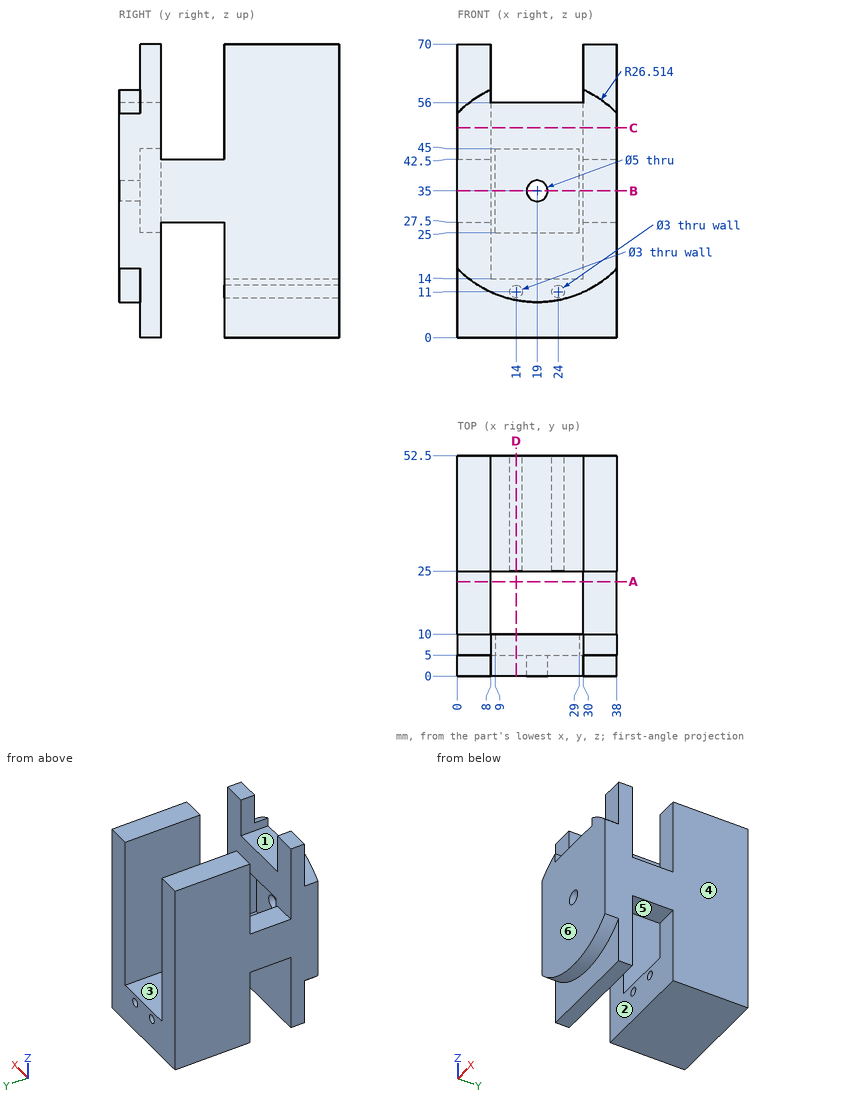
Geometry check sheet. Reference: drawing and pictorial views, mm from the part's lowest x, y, z. A direction names the side the tool comes from. Give positions to 0.01 mm unless a question says otherwise; leave off trailing zeros. Order: outer loops, then holes, each group sorted by start corner. A loop starts at its lowest first (then second) coordinate and runs counter-clockwise, first axis right, second up.
1. Access from +Z, -Z, +X, -X, +Y, -Y to the whole of each face (thin tool, end or side, straight path). Record for the marked faces 1, 2 and 3.
2. Section check C-C, the plane z = 50. Enter the section's corners in (x, y).
3. Section check A-A, the plane y = 22.5. Enter the section's corners in (x, z).
4. Section check D-D, the plane x = 14. Enter the section's corners in (y, z).
5. Thickness scan on L1, parallel to X at y = 33, z = 11; L2, parallel to X at y = 19, z = 38; L3, parallel to Y at x = 2.5, z = 66. Record the ranges inside material, lowest first.
6. Gauge pin test, flat ends, axial feed: pin 1 Ø5 at (x, z) = (34, 51.5) entering from -Y; pin 2 Ø1.5 at (x, z) = (13, 7) entering from -Y; pin 3 Ø4 at (x, y) = (23.5, 7.5) entering from +Z; pin 4 Ø2.5 at (x, z) = (24, 11) entering from +Y. Record the tip position at first contact, or that the pin passes through.
7. Section check B-B, the plane z = 35. Enter the section's corners in (x, y), and give its area (3 significant figures).
8. Release check for a two-part mould opening along Y. For the marked faces 4, 5 and 6 record: pulls with the +Y half, pulls with the -Y half, needs draft (parallel to the pull), parting line crosses it, or undercut.
Values follow:
1. face 1: +Z, +Y, -Y
1. face 2: -Z, +X, -X
1. face 3: +Z, +Y
2. outline: (0, 0) - (38, 0) - (38, 10) - (0, 10) - close; (0, 25) - (8, 25) - (8, 52.5) - (0, 52.5) - close; (30, 25) - (38, 25) - (38, 52.5) - (30, 52.5) - close
3. outline: (0, 27.5) - (8, 27.5) - (8, 42.5) - (0, 42.5) - close; (30, 27.5) - (38, 27.5) - (38, 42.5) - (30, 42.5) - close
4. outline: (0, 8.96) - (5, 8.96) - (5, 0) - (10, 0) - (10, 25) - (5, 25) - (5, 45) - (10, 45) - (10, 56) - (0, 56) - close; (25, 0) - (52.5, 0) - (52.5, 9.5) - (25, 9.5) - close; (25, 12.5) - (52.5, 12.5) - (52.5, 14) - (25, 14) - close
5. L1: x = 0 to 12.5, 15.5 to 22.5, 25.5 to 38
5. L2: x = 0 to 8, 30 to 38
5. L3: y = 5 to 10, 25 to 52.5
6. pin 1: stops at y = 0
6. pin 2: stops at y = 5
6. pin 3: stops at z = 56
6. pin 4: stops at y = 10
7. outline: (0, 0) - (16.5, 0) - (16.5, 5) - (9, 5) - (9, 10) - (8, 10) - (8, 52.5) - (0, 52.5) - close; (21.5, 0) - (38, 0) - (38, 52.5) - (30, 52.5) - (30, 10) - (29, 10) - (29, 5) - (21.5, 5) - close
7. area: 935 mm2
8. face 4: needs draft
8. face 5: undercut
8. face 6: pulls with the -Y half
